Autodesk Inventor part; units mm, degrees
ref_plane "YZ Plane" through (0, 0, 0) normal (1, 0, 0) x (0, 1, 0)
ref_plane "XZ Plane" through (0, 0, 0) normal (0, 1, 0) x (-1, 0, 0)
ref_plane "XY Plane" through (0, 0, 0) normal (0, 0, 1) x (1, 0, 0)
sketch "Sketch1" plane through (0, 0, 0) normal (0, 1, 0) x (-1, 0, 0)
  circle A0 centre (0, 0) radius 10.16
  dimension "d0" = 20.32
extrude "Extrusion1" add sketch "Sketch1" along normal blind 76.2
sketch "Sketch2" plane through (0, 76.2, 0) normal (0, 1, 0) x (1, 0, 0)
  circle A0 centre (0, 0) radius 19.05
  dimension "d3" = 38.1
extrude "Extrusion2" add sketch "Sketch2" along normal blind 12.7
sketch "Sketch6" plane through (0, 88.9, 0) normal (0, 1, 0) x (1, 0, 0)
  arc A0 (17.272, 0) -> (-17.272, 0) centre (0, 0) ccw
  line L0 (17.272, 0) -> (17.272, -8.0362)
  circle A1 centre (0, 0) radius 19.05
  line L1 (-17.272, 0) -> (-17.272, -8.5424)
  line L2 (17.272, -8.0362) -> (17.272, -33.241)
  line L3 (17.272, -33.241) -> (-17.272, -33.241)
  line L4 (-17.272, -33.241) -> (-17.272, -8.5424)
  dimension "d14" = 34.544
extrude "Extrusion5" cut sketch "Sketch6" against normal blind 9.525 contours L0 A1 L1 A0 | L2 L3 L4 L1 A1 picked at (0, -6.35)
sketch "Sketch7" plane through (0, 88.9, 0) normal (0, 1, 0) x (1, 0, 0)
  circle A0 centre (0, 0) radius 19.05
extrude "Extrusion6" add sketch "Sketch7" along normal blind 6.35
sketch "Sketch8" plane through (0, 95.25, 0) normal (0, 1, 0) x (1, 0, 0)
  circle A0 centre (0, 0) radius 9.779
  circle A1 centre (9.779, 0) radius 1.778
  circle A2 centre (0, -9.779) radius 1.778
  circle A3 centre (-9.779, 0) radius 1.778
  circle A4 centre (0, 9.779) radius 1.778
  dimension "d19" = 19.558
  dimension "d20" = 3.556
  dimension "d21" = 3.556
  dimension "d22" = 3.556
  dimension "d23" = 3.556
extrude "Extrusion7" cut sketch "Sketch8" against normal blind 6.35 contours A0 A1 | A0 A1 | A4 A0 | A0 A4 | A2 A0 | A0 A2 | A3 A0 | A0 A3
sketch "Sketch9" plane through (0, 95.25, 0) normal (0, 1, 0) x (1, 0, 0)
  circle A0 centre (0, 0) radius 10.16
  circle A1 centre (0, 0) radius 3.2004
  dimension "d26" = 6.4008
extrude "Extrusion8" cut sketch "Sketch9" against normal through all contours A1
sketch "Sketch10" plane through (0, 0, 0) normal (0, -1, 0) x (1, 0, 0)
  circle A0 centre (0, 0) radius 12.7
  circle A1 centre (0, 0) radius 3.2004
  dimension "d29" = 25.4
extrude "Extrusion9" add sketch "Sketch10" along normal blind 6.35
properties part number "Rotating1inPart"
Could you check a few things on this model? Use its own coordinates, in mm. A direction names the side the tool comes from. Give positions to 0.01 mm unless a question says otherwise; leave off trailing zeros. Order: outer loops, then holes, each group sorted by start corner. A loop starts at its lowest first (then second) coordinate and runs counter-clockwise, first axis right, second up.
Q1. Suppose I cut it at C-C, the plane x = -15. Write out the boundary of the cut face in (y, z) (3 decimals), and give its area (3 significant figures).
Q2. For faces 1 (the flat face through (-6, 0, 9)), 2 (the cylindrical face through (0.38, 84.204, -17.268)), 3 (the cylindrical face through (-2.75, -3.13, 12.4)), 4 (the flat face through (3, -6.35, -3)), 5 (the cylindrical face through (-0.385, 92.119, 11.515)), which set-ups out of +Z, -Z, +X, -X, +Y, -Y let a thin tool reach every point of the face, with its end or its side?
Q3. Suppose I cut it at B-B, the plane y = 77.5. Write out the boundary of the cut face in (x, z).
Q4. Suppose I cut it at D-D, the plane y = 21.5. Write out the boundary of the cut face in (x, z).
Q5. Suppose I cut it at A-A, the plane x = 0. Count the separate pieces of the cut face and the enclosed holes in it, and give its area (4 significant figures).
Q6. We'd pull the mould along X, two halves only. Please class faces 6 (the cylindrical face through (1.323, 37.567, -10.074)), 7 (the flat face through (4, 95.25, 0)), 8 (the cylindrical face through (0, 92, -8)), 9 (the flat face through (17.272, 84, 4)): +X half, -X half, draft (parallel to the pull), parting line (faces both ways), or undercut.
Q7. I'm going to push flat-ended pins straight in: P1, Ø3, axis at x = 0, z = -9.779, coming from the +Y side (3 decimals); P2, Ø4, axis at y = 83, z = 6, coming from the -X side; P3, Ø4, axis at x = -7.5, y = 29.5, coming from the +Z side. Where does each tip first touch, or does it pass through?
Q8. If I drill on line 1 along X through (y, z) = (92.75, 0); line 2 along Y through (x, z) = (8.5, -9) (3 decimals), over which ranges is the centre line in solid material (lowest first)?
Solution:
1. outline: (76.2, -11.743) - (95.25, -11.743) - (95.25, 11.743) - (88.9, 11.743) - (88.9, -8.563) - (79.375, -8.563) - (79.375, 11.743) - (76.2, 11.743) - close
1. area: 254 mm2
2. face 1: none
2. face 2: +Z
2. face 3: -Y
2. face 4: +Z, -Z, +X, -X, -Y
2. face 5: +Y
3. outline: circle Ø38.1 at (0, 0); hole circle Ø6.4 at (0, 0)
4. outline: circle Ø20.32 at (0, 0); hole circle Ø6.4 at (0, 0)
5. separate pieces: 5
5. enclosed holes: 0
5. area: 1,455 mm2
6. face 6: parting line
6. face 7: draft
6. face 8: undercut
6. face 9: undercut
7. P1: stops at y = 79.375
7. P2: stops at x = -18.63
7. P3: stops at z = 8.54
8. line 1: x = -19.05 to -11.56, -8 to -3.2, 3.2 to 8, 11.56 to 19.05
8. line 2: y = -6.35 to 0, 76.2 to 79.375, 88.9 to 95.25
